```python
from build123d import *

# Parameters (mm, degrees)
SKETCH1_R           = 12.5
BOSS_EXTRUDE1_DEPTH = 500
SKETCH3_R           = 15
BOSS_EXTRUDE2_DEPTH = 25
FILLET2_R           = 5
SHELL1_T            = -1


with BuildPart() as part:
    # Sketch1 → Boss-Extrude1 (new body)
    with BuildSketch(Plane(origin=(0, 0, 0), x_dir=(1, 0, 0), z_dir=(0, 1, 0))):
        with Locations(Location((0, 0, 0), (0, 0, 270))):
            Circle(SKETCH1_R)
    extrude(amount=BOSS_EXTRUDE1_DEPTH)

    # Sketch3 → Boss-Extrude2 (add)
    with BuildSketch(Plane.XZ):
        with Locations(Location((0, 0, 0), (0, 0, 270))):
            Circle(SKETCH3_R)
    extrude(amount=-BOSS_EXTRUDE2_DEPTH)

    # Fillet2
    fillet2_edges = [part.edges().sort_by_distance(p)[0] for p in [
        (0, 0, 15),
    ]]
    fillet(fillet2_edges, radius=FILLET2_R)

    # Shell1
    shell1_openings = [part.faces().sort_by_distance(p)[0] for p in [
        (0, 500, 0),
    ]]
    offset(amount=SHELL1_T, openings=shell1_openings, kind=Kind.INTERSECTION)


solid = part.part
```
Build history of the part. All positions in model axes, mm. A direction names the side the tool comes from. Round coordinates to 2 decimals unless told otherwise and drop trailing zeros. Order: outer loops, then holes, each group sorted by start corner. A loop starts at its lowest first (then second) coordinate and runs counter-clockwise, first axis right, second up. Notation, with made-up numbers: (21.5, 40) -> (75.5, 40) arc R37 ccw to (75.5, 77) -> close; hole circle Ø7 at (71.5, 88). An arc over 180 degrees is marked (long way). Answer in a Markdown table with one row per item.
1) Which spindle directions (+Z, -Z, +X, -X, +Y, -Y) get a long thin tool onto all of the face, cutting with end or side? Do faces 1 (the flat face through (0, 0, 0)), 2 (the flat face through (11.5, 24, 2.1)), 3 (the flat face through (12.3, 25, 3.4)). Say none if no direction does.
Values:
| item | result |
|---|---|
| face 1 | +Z, -Z, +X, -X, -Y |
| face 2 | none |
| face 3 | +Y |
2) Band-saw the part on B-B on z = 0. Give the cut face in (x, y), and give its area (3 significant figures).
Values:
| item | result |
|---|---|
| outline | (-15, 5) arc R5 ccw to (-10, 0) -> (10, 0) arc R5 ccw to (15, 5) -> (15, 25) -> (12.5, 25) -> (12.5, 500) -> (11.5, 500) -> (11.5, 24) -> (14, 24) -> (14, 5) arc R4 cw to (10, 1) -> (-10, 1) arc R4 cw to (-14, 5) -> (-14, 24) -> (-11.5, 24) -> (-11.5, 500) -> (-12.5, 500) -> (-12.5, 25) -> (-15, 25) -> close |
| area | 1,030 mm2 |
3) Mould opens along X. For faces 4 (the cylindrical face through (9.7, 258.67, 6.18)), 5 (the cylindrical face through (3.755, 259.175, 11.923)), 6 (the flat face through (-11, 500, 4)) say: released by +X, released by -X, zero draft, split by the parting line, or undercut.
Values:
| item | result |
|---|---|
| face 4 | undercut |
| face 5 | split by the parting line |
| face 6 | zero draft |
4) Pin check, flat tips, straight feed: P1, Ø6, axis at x = -10, y = 244, coming from the +Z side; P2, Ø6, axis at x = 1, y = 52, coming from the -Z side; P3, Ø8, axis at x = 6, y = 144, coming from the -Z side. Stop position of each tip, or through.
Values:
| item | result |
|---|---|
| P1 | z = 10.36 |
| P2 | z = -12.5 |
| P3 | z = -12.34 |
5) Wall check: L1, parallel to Z at x = 1.25, y = 404; L2, parallel to X at y = 264, z = 0. Give the ranges that are in metal, low to high.
Values:
| item | result |
|---|---|
| L1 | -12.44 to -11.43, 11.43 to 12.44 |
| L2 | -12.5 to -11.5, 11.5 to 12.5 |
6) Band-saw the part on C-C on y = 227. Give the cut face in (x, z), and give its area (3 significant figures).
Values:
| item | result |
|---|---|
| outline | circle Ø25 at (0, 0); hole circle Ø23 at (0, 0) |
| area | 75.4 mm2 |
7) Band-saw the part on A-A on x = 0. Give the cut face in (y, z).
Values:
| item | result |
|---|---|
| outline | (0, -10) arc R5 ccw to (5, -15) -> (25, -15) -> (25, -12.5) -> (500, -12.5) -> (500, -11.5) -> (24, -11.5) -> (24, -14) -> (5, -14) arc R4 cw to (1, -10) -> (1, 10) arc R4 cw to (5, 14) -> (24, 14) -> (24, 11.5) -> (500, 11.5) -> (500, 12.5) -> (25, 12.5) -> (25, 15) -> (5, 15) arc R5 ccw to (0, 10) -> close |
